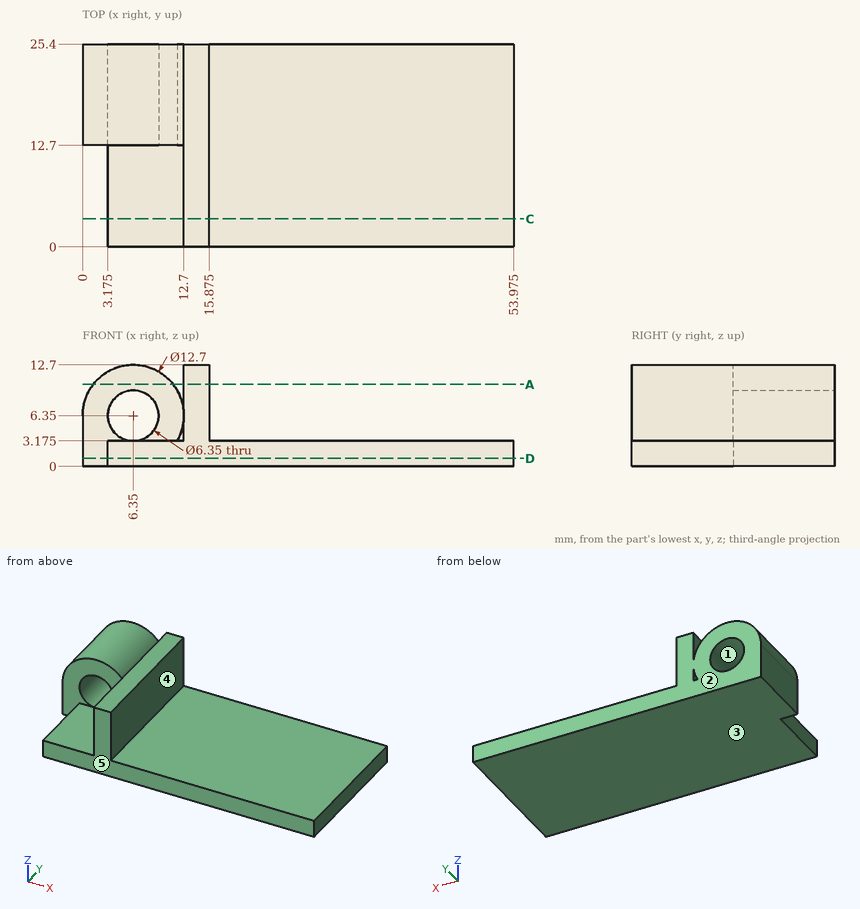
Geometry check sheet. Reference: drawing and pictorial views, mm from the part's lowest x, y, z. A direction names the side the tool comes from. Give positions to 0.01 mm unless a question says otherwise; leave off trailing zeros. Write each loop counter-clockwise with the first axis right and the second up, starting at its lowest first coordinate (ties: lowest second). Pieces come first, ordered by that corner, then holes. Notation, with made-up numbers: M 9,-32.75 L 67,-32.75 A11 ccw 67,-16.75 Z; hole C 60.25,77.5 d1. An arc over 180 degrees is marked long. Put each result on its own line as item: value. Start each with the question number.
1. Set-up check for the marked faces 4 and 5: record each of +Z, -Z, +X, -X, +Y, -Y from which the full face is reachable in a straight line by a thin tool's end or side.
2. Section check D-D (z = 1). Record the cut outline in (x, y) (3 decimals).
3. Section check A-A (z = 10.25). Record the cut outline in (x, y) (3 decimals), and give its area (3 significant figures).
4. Scan lines: line 1 along Z through (x, y) = (6.35, 19.75) (3 decimals); line 2 along X through (y, z) = (4, 9.5) (3 decimals); line 3 along X through (y, z) = (9.5, 1.5) (3 decimals). Record each from-to range of solid material in increasing order. Write a range as [from, to].
5. Section check C-C (y = 3.5). Record the cut outline in (x, z) (3 decimals).
6. Draft check along Z on the marked faces 1, 2 and 3. Enter one of: +Z half, -Z half, draft (parallel to the pull), parting line (faces both ways), or undercut.
7. Go/stop test with flat-tipped pins: pin 1 Ø6 at (y, z) = (17, 8) entering from +X (3 decimals); pin 2 Ø5 at (y, z) = (10, 9.5) entering from -X; pin 3 Ø7.5 at (x, y) = (30, 12.5) entering from +Z (3 decimals); pin 4 Ø5 at (y, z) = (21.5, 2) entering from -X. Record where each tip stops, or that it passes through.
Answer list:
1. face 4: +Z, +X, +Y, -Y
1. face 5: +Z, -Z, +X, -X, -Y
2. outline: M 0,12.7 L 3.175,12.7 L 3.175,0 L 53.975,0 L 53.975,25.4 L 0,25.4 Z
3. outline: M 1.339,12.7 L 11.361,12.7 L 11.361,25.4 L 1.339,25.4 Z; M 12.7,0 L 15.875,0 L 15.875,25.4 L 12.7,25.4 Z
3. area: 208 mm2
4. line 1: [0, 3.175], [9.525, 12.7]
4. line 2: [12.7, 15.875]
4. line 3: [3.175, 53.975]
5. outline: M 3.175,0 L 53.975,0 L 53.975,3.175 L 15.875,3.175 L 15.875,12.7 L 12.7,12.7 L 12.7,3.175 L 3.175,3.175 Z
6. face 1: undercut
6. face 2: draft
6. face 3: -Z half
7. pin 1: x = 15.875
7. pin 2: x = 12.7
7. pin 3: z = 3.175
7. pin 4: x = 0
